Could you check a few things on this model? Use its own coordinates, in mm. A direction names the side the tool comes from. Give positions to 0.01 mm unless a question says otherwise; leave off trailing zeros. Order: outer loops, then holes, each group sorted by start corner. A loop starts at its lowest first (then second) coordinate and runs counter-clockwise, first axis right, second up. Notation, with made-up numbers: (30, -38.5) - (60, -38.5) arc R9 ccw to (60, -26.5) - close; hole circle Ø5 at (-33.75, 4.25). An arc over 180 degrees is marked (long way). One line per question, with ' | ' between items. Start each with the question number.
1. Imagine slicing it at D-D (x = -2.2). Please give me the cut outline in (y, z), and give its area (3 significant figures).
2. Imagine slicing it at B-B (y = 5.25). Please give me the cut outline in (x, z).
3. Which directions (+Z, -Z, +X, -X, +Y, -Y) give clear straight access to the entire face, cutting with the end or side of a thin tool? Please do faces 1 (the flat face through (2, 2.5, 0)), 2 (the flat face through (-2, 2.5, 0)), 3 (the cylindrical face through (-1.34, 3.25, -2.11)).
4. I need wall thicknesses on probe 1 along X at (y, z) = (4.75, -0.1); probe 2 along Y at (x, z) = (2.1, -0.3); probe 3 along Z at (x, y) = (-1.3, 0.75). Which ranges of each line are inside material? Lowest first, please. Write a range as from..to.
5. Imagine slicing it at A-A (z = 0). Please give me the cut outline in (x, y), and give its area (3 significant figures).
6. For P1, Ø1.2, axis at y = 4, z = 0, coming from the -X side; P2, Ø3, axis at y = 4.5, z = 0.5, coming from the +X side; P3, Ø0.5, axis at x = 2, z = 0, coming from the +Y side, each with a flat end and sliding along its axis, tell me the tip position at first contact or that it passes through.
7. Imagine slicing it at C-C (z = -0.95). Please give me the cut outline in (x, y), and give its area (3 significant figures).
Autodesk Inventor part; units mm, degrees
ref_plane "YZ Plane" through (0, 0, 0) normal (1, 0, 0) x (0, 1, 0)
ref_plane "XZ Plane" through (0, 0, 0) normal (0, 1, 0) x (-1, 0, 0)
ref_plane "XY Plane" through (0, 0, 0) normal (0, 0, 1) x (1, 0, 0)
sketch "Sketch1" plane through (0, 0, 0) normal (0, 1, 0) x (-1, 0, 0)
  circle A0 centre (0, 0) radius 2.5
  dimension "d0" = 5
extrude "Extrusion1" add sketch "Sketch1" along normal blind 2.5
sketch "Sketch2" plane through (0, 2.5, 0) normal (0, 1, 0) x (1, 0, 0)
  circle A0 centre (0, 0) radius 2.5
  line L0 (1.5, -2) -> (-1.5, -2)
  line L1 (-1.5, -2) -> (-1.5, 2)
  line L2 (-1.5, 2) -> (1.5, 2)
  line L3 (1.5, 2) -> (1.5, -2)
  line L4 (1.5, -2) -> (-1.5, 2) construction
  line L5 (-1.5, -2) -> (1.5, 2) construction
  arc A1 (-1.5, -2) -> (1.5, -2) centre (0, 0) ccw
  arc A2 (-1.5, 2) -> (-1.5, -2) centre (0, 0) ccw
  arc A3 (1.5, 2) -> (-1.5, 2) centre (0, 0) ccw
  arc A4 (1.5, -2) -> (1.5, 2) centre (0, 0) ccw
  dimension "d3" = 3
extrude "Extrusion2" add sketch "Sketch2" along normal blind 6 contours L2 A0 | L3 L0 L1 L2 | A0 L0
properties part number "small_stepper_shaft"
Results found:
1) outline: (0, -1.19) - (2.5, -1.19) - (2.5, 1.19) - (0, 1.19) - close | area: 5.94 mm2
2) outline: (-1.5, -2) arc R2.5 ccw to (1.5, -2) - (1.5, 2) arc R2.5 ccw to (-1.5, 2) - close
3) face 1: +Z, -Z, +X, +Y | face 2: +Z, -Z, -X, +Y | face 3: +Y, -Y
4) probe 1: x = -1.5..1.5 | probe 2: y = 0..2.5 | probe 3: z = -2.14..2.14
5) outline: (-2.5, 0) - (2.5, 0) - (2.5, 2.5) - (1.5, 2.5) - (1.5, 8.5) - (-1.5, 8.5) - (-1.5, 2.5) - (-2.5, 2.5) - close | area: 30.5 mm2
6) P1: stops at x = -1.5 | P2: stops at x = 1.5 | P3: stops at y = 2.5
7) outline: (-2.31, 0) - (2.31, 0) - (2.31, 2.5) - (1.5, 2.5) - (1.5, 8.5) - (-1.5, 8.5) - (-1.5, 2.5) - (-2.31, 2.5) - close | area: 29.6 mm2
